Geometry check sheet. Reference: the model listing, model coordinates, mm. Face numbers are marked on the shaded views. Round coordinates to 2 decimals unless told otherwise and drop trailing zeros. Write each loop counter-clockwise with the first axis right and the second up, starting at its lowest first coordinate (ties: lowest second). Pieces come first, ordered by that corner, then holes. Notation, with made-up numbers: (82.5, 45) -> (89.5, 45) arc R19 ccw to (89.5, 66) -> close; hole circle Ø3 at (22, 28.25). An arc over 180 degrees is marked (long way). One line per question, with ' | ' between items.
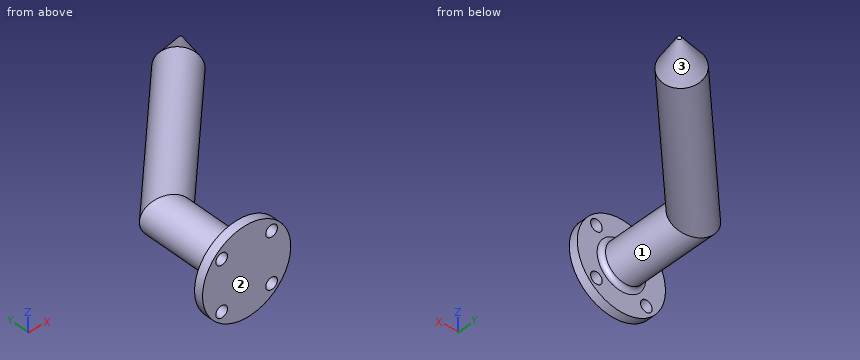
Autodesk Inventor part; units mm, degrees
ref_plane "Work Plane1" through (84.8528, 134.8528, 0) normal (0.7071068, 0.7071068, 0) x (-0.7071068, 0.7071068, 0)
ref_plane "YZ Plane" through (0, 0, 0) normal (1, 0, 0) x (0, 1, 0)
ref_plane "XZ Plane" through (0, 0, 0) normal (0, 1, 0) x (-1, 0, 0)
sketch "Sketch1" plane through (0, 0, 0) normal (0, 0, 1) x (1, 0, 0)
  line L0 (0, 0) -> (0, 50)
  line L1 (0, 50) -> (70.7107, 120.7107)
  line L2 (0, 50) -> (30.994, 50) construction
  line L3 (70.7107, 120.7107) -> (84.8528, 134.8528) construction
  dimension "d0" = 50
  dimension "d1" = 100
  dimension "d2" = 45
  dimension "d24" = 120
sketch "Sketch2" plane through (0, 0, 0) normal (0, 1, 0) x (-1, 0, 0)
  circle A0 centre (0, 0) radius 11.25
  circle A1 centre (0, 0) radius 8.75 construction
  dimension "d6" = 17.5
  dimension "d7" = 2.5
  dimension "d27" = 22.5
sweep "Sweep1" add profiles "Sketch2" path "Sketch1"
sketch "Sketch3" plane through (0, 0, 0) normal (0, 1, 0) x (-1, 0, 0)
  circle A0 centre (0, 0) radius 11.25
  circle A1 centre (0, 0) radius 20 construction
  circle A2 centre (0, 0) radius 25
  dimension "d8" = 40
  dimension "d9" = 5
  dimension "d10" = 50
extrude "Extrusion1" add sketch "Sketch3" along normal blind 5
sketch "Sketch4" plane through (0, 5, 0) normal (0, 1, 0) x (1, 0, 0)
  circle A0 centre (0, 0) radius 20 construction
  point P0 (-14.1421, 14.1421)
  point P1 (-14.1421, -14.1421)
  point P2 (14.1421, -14.1421)
  point P3 (14.1421, 14.1421)
hole "Hole1" at (-14.1421, 5, -14.1421) at (14.1421, 5, -14.1421) at (-14.1421, 5, 14.1421) at (14.1421, 5, 14.1421) direction (0, -1, 0) diameter 6.6 end through all
fillet "Fillet1" radius 2.5 1 edges at (11.25, 5, 0)
ref_plane "Work Plane1" through (84.8528, 134.8528, 0) normal (0.7071068, 0.7071068, 0) x (-0.7071068, 0.7071068, 0)
sketch "Sketch8" plane through (84.8528, 134.8528, 0) normal (0.7071068, 0.7071068, 0) x (-0.7071068, 0.7071068, 0)
  circle A0 centre (0, 0) radius 1
  point P0 (-35.3553, 0)
  dimension "d34" = 2
loft "Loft2" add profiles "Sketch8" section 1 edges at (78.6656, 112.7557, 0)
properties part number "Herramienta1-2" material "PLA"
(1) Sectioned sample at A-A on z = 15.5. Record the cut outline in (x, y), then the cut area to 3 significant figures.
Resolved:
outline: (-19.62, 0) -> (-17.15, 0) -> (-17.15, 5) -> (-19.62, 5) -> close; (-11.13, 0) -> (11.13, 0) -> (11.13, 5) -> (-11.13, 5) -> close; (17.15, 0) -> (19.62, 0) -> (19.62, 5) -> (17.15, 5) -> close | area: 136 mm2
(2) Material ranges on line 1 (Y direction, x = -12, z = -10); line 2 (Z direction, x = 0, y = 9.5); line 3 (X direction, y = 100, z = -5), recorded low to high.
Resolved:
line 1: y = 0 to 5 | line 2: z = -11.25 to 11.25 | line 3: x = 35.75 to 64.25
(3) Draft check along Y on the marked faces 1, 2 and 3. Enter one of: +Y half, -Y half, draft (parallel to the pull), parting line (faces both ways), or undercut.
Resolved:
face 1: undercut | face 2: -Y half | face 3: parting line
(4) Go/stop test with flat-tipped pins: pin 1 (8 mm diameter, centred on y = 119.5, z = -6, fed in from -X); pin 2 (5 mm diameter, centred on y = 39, z = -8, fed in from -X); pin 3 (1 mm diameter, centred on y = 94.5, z = 8.5, fed in from -X); pin 4 (8.5 mm diameter, centred on x = 14.14, z = 14.14, fed in from -Y). Record where each tip stops, or that it passes through.
Resolved:
pin 1: stops at x = 51.16 | pin 2: stops at x = -9.81 | pin 3: stops at x = 33.16 | pin 4: stops at y = 0
(5) Sectioned sample at B-B on y = 31. Record the cut outline in (x, z).
Resolved:
outline: circle Ø22.5 at (0, 0)
(6) Sectioned sample at C-C on z = -21.5. Record the cut outline in (x, y), then the cut area to 3 significant figures.
Resolved:
outline: (-12.76, 0) -> (12.76, 0) -> (12.76, 5) -> (-12.76, 5) -> close | area: 128 mm2
